```python
from build123d import *

# Parameters (mm, degrees)
EXTRUDE_1_DEPTH = 480
SCALE_1_SCALE   = 1.3


with BuildPart() as part:
    # 草图1 → 凸台-拉伸1 (new body)
    with BuildSketch(Plane.XY):
        with BuildLine():
            Line((-7368.547684402, 5393.3126292), (-7227.479223851, 5199.14855055))
            ThreePointArc((-7227.479223851, 5199.14855055), (-7002.704039562, 5336.890960636), (-6759.14855055, 5437.774947376))
            Line((-6759.14855055, 5437.774947376), (-6833.3126292, 5666.028511287))
            ThreePointArc((-6833.3126292, 5666.028511287), (-6989.477063432, 5607.677609574), (-7139.991111067, 5536))
            ThreePointArc((-7139.991111067, 5536), (-7256.775458313, 5468.670521429), (-7368.547684402, 5393.3126292))
        make_face()
    extrude(amount=EXTRUDE_1_DEPTH)


with BuildPart() as part_1:
    # 缩放比例1: scaled about (0, 0, 0)
    add(part.part.scale(SCALE_1_SCALE))


solid = part_1.part
```
Geometry: final body of the model. Coordinates: model frame, mm. Coordinates: 2 decimals unless noted, no trailing zeros. Loops run counter-clockwise (first coordinate to the right, second up) from the corner with the lowest first, then second, coordinate; pieces in that order, holes last. Notation, with made-up numbers: (43, -31.5) -> (85, -31.5) arc R14 ccw to (85, -23.5) -> close; hole circle Ø3 at (89, 79.25). An arc over 180 degrees is marked (long way). Use a Markdown table: item, result. Add a question column.
(1) Line query: line 1 along X through (y, z) = (6937.5, 198.5); line 2 along X through (y, z) = (6999, 110); line 3 along Y through (x, z) = (-9409.5, 503). Output: solid intervals per line, ascending.
(2) Section query A-A, the plane z = 289.5. Return loops of the section in (x, y).
(3) Section query C-C, the plane y = 7270. Return loops of the section in (x, z).
(4) Pin query (flat end, axial travel): pin 1 Ø6 at (y, z) = (6963, 202) entering from -X; pin 2 Ø3 at (x, z) = (-9025.5, 176.5) entering from +Y; pin 3 Ø4 at (y, z) = (7106, 400) entering from +X; pin 4 Ø1 at (x, y) = (-9335.5, 7109) entering from -Z. Return the tip coordinate at first contact, or that it passes through.
(5) Section query B-B, the plane x = -8957.5. Return loops of the section in (y, z).
Answer:
| question | item | result |
|---|---|---|
| 1 | line 1 | x = -9525.49 to -9104.41 |
| 1 | line 2 | x = -9570.17 to -8973.28 |
| 1 | line 3 | y = 6777.86 to 7124.25 |
| 2 | outline | (-9579.11, 7011.31) -> (-9395.72, 6758.89) arc R2184 cw to (-8786.89, 7069.11) -> (-8883.31, 7365.84) arc R2496 ccw to start |
| 3 | outline | (-9132.16, 0) -> (-8852.17, 0) -> (-8852.17, 624) -> (-9132.16, 624) -> close |
| 4 | pin 1 | stops at x = -9546.19 |
| 4 | pin 2 | stops at y = 7315.42 |
| 4 | pin 3 | stops at x = -8798.23 |
| 4 | pin 4 | stops at z = 0 |
| 5 | outline | (7005.7, 0) -> (7340.43, 0) -> (7340.43, 624) -> (7005.7, 624) -> close |
